from build123d import *

# Parameters (mm, degrees)
F0_W     = 133.35
F0_H     = 82.55
F0_W_2   = 124.46
F0_H_2   = 73.66
F0_W_3   = 118.11
F0_H_3   = 67.31
F1_DEPTH = 6.35
F2_DEPTH = 9.525
F3_R     = 1.27


with BuildPart() as f1:
    # F0 (on Front) → F1 (new body)
    with BuildSketch(Plane.XZ):
        Rectangle(F0_W, F0_H)
        Rectangle(F0_W_2, F0_H_2, mode=Mode.SUBTRACT)
        Rectangle(F0_W_2, F0_H_2)
        Rectangle(F0_W_3, F0_H_3, mode=Mode.SUBTRACT)
        Rectangle(F0_W_3, F0_H_3)
    extrude(amount=F1_DEPTH)

    # F0 (on Front) → F2 (join)
    with BuildSketch(Plane.XZ):
        Rectangle(F0_W_2, F0_H_2)
        Rectangle(F0_W_3, F0_H_3, mode=Mode.SUBTRACT)
    extrude(amount=F2_DEPTH)

    # F3
    f3_edges = [f1.edges().sort_by_distance(p)[0] for p in [
        (0, 0, -41.275),
        (-66.675, 0, 0),
        (-66.675, -3.175, -41.275),
        (-66.675, -3.175, 41.275),
        (0, 0, 41.275),
        (66.675, -3.175, 41.275),
        (66.675, 0, 0),
        (66.675, -3.175, -41.275),
    ]]
    fillet(f3_edges, radius=F3_R)


solid = f1.part
Build history of the part. All positions in model axes, mm. A direction names the side the tool comes from. Give positions to 0.01 mm unless a question says otherwise; leave off trailing zeros. Order: outer loops, then holes, each group sorted by start corner. A loop starts at its lowest first (then second) coordinate and runs counter-clockwise, first axis right, second up. Notation, with made-up numbers: M 19.5,44 L 29.5,44 A30 ccw 29.5,76 Z; hole C 70,25.5 d2. An arc over 180 degrees is marked long. Put each result on its own line as item: value.
Item 1: Drop flat-ended pins along their axis: pin 1 Ø1.6 at (y, z) = (-8, 14.5) entering from +X; pin 2 Ø1.6 at (x, y) = (28, -7) entering from +Z (3 decimals); pin 3 Ø12 at (x, z) = (-20.5, 13) entering from -Y; pin 4 Ø2.5 at (x, y) = (21.5, -8) entering from -Z. Give the stop position or say it passes through.
Results are:
pin 1: x = 62.23
pin 2: z = 41.275
pin 3: y = -6.35
pin 4: z = -36.83
Item 2: Which spindle directions (+Z, -Z, +X, -X, +Y, -Y) get a long thin tool onto all of the face, cutting with end or side? Do faces 1 (the face through (-1, -8, -36.83)), 2 (the face through (-1, -8, 36.83)), 3 (the face through (-62.23, -8, -1)), 4 (the face through (-1, -8, 33.655)). Say none if no direction does.
Results are:
face 1: -Z, +X, -X, -Y
face 2: +Z, +X, -X, -Y
face 3: +Z, -Z, -X, -Y
face 4: -Y
Item 3: Cut at A-A on z = -17.5. Write the cut outline in (x, y) (3 decimals).
Results are:
outline: M -66.675,-6.35 L -62.23,-6.35 L -62.23,-9.525 L -59.055,-9.525 L -59.055,-6.35 L 59.055,-6.35 L 59.055,-9.525 L 62.23,-9.525 L 62.23,-6.35 L 66.675,-6.35 L 66.675,-1.27 A1.27 ccw 65.405,0 L -65.405,0 A1.27 ccw -66.675,-1.27 Z
Item 4: Cut at B-B on y = -8. Write the cut outline in (x, z) (3 decimals).
Results are:
outline: M -62.23,-36.83 L 62.23,-36.83 L 62.23,36.83 L -62.23,36.83 Z; hole M -59.055,-33.655 L 59.055,-33.655 L 59.055,33.655 L -59.055,33.655 Z
Item 5: Pull direction X, two halves, no side cores. Call faces 5 (the face through (62.23, -8, -1)), 6 (the face through (-1, -4, 41.275)), 7 (the face through (-59.055, -8, 0)): +X half, -X half, draft (parallel to the pull), parting line (faces both ways), or undercut.
Results are:
face 5: +X half
face 6: draft
face 7: undercut
Item 6: Cut at C-C on x = 20.5. Write the cut outline in (y, z) (3 decimals).
Results are:
outline: M -9.525,-36.83 L -6.35,-36.83 L -6.35,-41.275 L -1.27,-41.275 A1.27 ccw 0,-40.005 L 0,40.005 A1.27 ccw -1.27,41.275 L -6.35,41.275 L -6.35,36.83 L -9.525,36.83 L -9.525,33.655 L -6.35,33.655 L -6.35,-33.655 L -9.525,-33.655 Z
Item 7: Wall check: probe 1 along Z at (x, y) = (-42, -8.75) (3 decimals); probe 2 along X at (y, z) = (-9, -16) (3 decimals); probe 3 along Y at (x, z) = (30, 23.5). Give the ranges that are in metal, low to high.
Results are:
probe 1: -36.83 to -33.655, 33.655 to 36.83
probe 2: -62.23 to -59.055, 59.055 to 62.23
probe 3: -6.35 to 0
